Geometry: final body of the model. Coordinates: model frame, mm. A direction names the side the tool comes from. Give positions to 0.01 mm unless a question says otherwise; leave off trailing zeros. Order: outer loops, then holes, each group sorted by start corner. A loop starts at its lowest first (then second) coordinate and runs counter-clockwise, first axis right, second up. Notation, with made-up numbers: (17, 35) -> (26, 35) arc R12 cw to (26, 40) -> close; hole circle Ø1 at (61.5, -22). An arc over 180 degrees is marked (long way). Write item = value, one per line.
```python
from build123d import *

# Parameters (mm, degrees)
F0_W      = 32.2
F0_H      = 31.2
F1_DEPTH  = 4.2
F2_W      = 9.2
F2_H      = 8.6
F3_DEPTH  = 8.4
F2_W_2    = 25.4
F2_H_2    = 24.4
F4_DEPTH  = 4.5
F5_DEPTH  = 5
F2_W_3    = 17
F2_H_3    = 2
F6_DEPTH  = 4.1
F7_DEPTH  = 6.8
F8_R      = 2.5
F9_DEPTH  = 2
F10_R     = 2.5
F11_DEPTH = 2


with BuildPart() as f1:
    # F0 (on Front) → F1 (new body, symmetric)
    with BuildSketch(Plane.XZ):
        Rectangle(F0_W, F0_H)
    extrude(amount=F1_DEPTH, both=True)

    # F2 (on face) → F3 (cut, through all)
    with BuildSketch(Plane.XZ.offset(4.2)):
        with Locations((0, -2.8)):
            Rectangle(F2_W, F2_H)
    extrude(amount=-F3_DEPTH, mode=Mode.SUBTRACT)

    # F2 (on face) → F4 (cut)
    with BuildSketch(Plane.XZ.offset(4.2)):
        Polygon((14.1, -13.6), (14.1, 13.6), (-14.1, 13.6), (-14.1, -13.6), (-8.5, -13.6), (8.5, -13.6), align=None)
        Rectangle(F2_W_2, F2_H_2, mode=Mode.SUBTRACT)
    extrude(amount=-F4_DEPTH, mode=Mode.SUBTRACT)

    # F5 (cut): a face of the model
    f5_faces = [f1.faces().sort_by_distance(p)[0] for p in [
        (-12.3477898355, -4.2, 0),
    ]]
    extrude(f5_faces, amount=-F5_DEPTH, mode=Mode.SUBTRACT)

    # F2 (on face) → F6 (cut)
    with BuildSketch(Plane.XZ.offset(4.2)):
        with Locations((0, -14.6)):
            Rectangle(F2_W_3, F2_H_3)
    extrude(amount=-F6_DEPTH, mode=Mode.SUBTRACT)

    # F2 (on face) → F7 (cut)
    with BuildSketch(Plane.XZ.offset(4.2)):
        Polygon((-7.1, 1.5), (-4.6, 1.5), (4.6, 1.5), (7.1, 1.5), (7.1, 9.7), (-7.1, 9.7), align=None)
    extrude(amount=-F7_DEPTH, mode=Mode.SUBTRACT)

    # F8 (on face) → F9 (cut)
    with BuildSketch(Plane.YZ.offset(16.1)):
        with Locations((0, -10.6)):
            Circle(F8_R)
    extrude(amount=-F9_DEPTH, mode=Mode.SUBTRACT)

    # F10 (on face) → F11 (cut)
    with BuildSketch(Plane(origin=(-16.1, 0, 0), x_dir=(0, -1, 0), z_dir=(-1, 0, 0))):
        with Locations((0, -10.6)):
            Circle(F10_R)
    extrude(amount=-F11_DEPTH, mode=Mode.SUBTRACT)


solid = f1.part
```
1) Reachability of faces 4 (the face through (0, 2, 9.7)), 5 (the face through (0, -0.1, -15)), 6 (the face through (-4.6, 2, -3)) from +Z, -Z, +X, -X, +Y, -Y: full face, straight path, thin tool, end or side. Return the list, or none.
Check sheet entries:
face_4 = -Y
face_5 = -Z, -Y
face_6 = +Y, -Y
2) Section query C-C (z = -10.6). Output: boundary loops of the cut face in (x, y), plus the area to 3 significant figures.
Check sheet entries:
outline = (-16.1, -4.2) -> (-14.1, -4.2) -> (-14.1, -2.5) -> (-16.1, -2.5) -> close; (-16.1, 2.5) -> (-14.1, 2.5) -> (-14.1, 0.3) -> (-12.7, 0.3) -> (-12.7, 0.8) -> (12.7, 0.8) -> (12.7, 0.3) -> (14.1, 0.3) -> (14.1, 2.5) -> (16.1, 2.5) -> (16.1, 4.2) -> (-16.1, 4.2) -> close; (14.1, -4.2) -> (16.1, -4.2) -> (16.1, -2.5) -> (14.1, -2.5) -> close
area = 111 mm²
3) First-contact query: P1, Ø2, axis at x = 2.5, z = -14, coming from the -Y side; P2, Ø4, axis at y = 0, z = -10.6, coming from the -X side; P3, Ø2, axis at x = 0, z = 2, coming from the -Y side. Flat tips, straight axial feed; report the tip coordinate or a pass-through.
Check sheet entries:
P1 = -0.1
P2 = -14.1
P3 = 2.6
4) Section query B-B (x = 1). Output: boundary loops of the cut face in (y, z).
Check sheet entries:
outline = (-4.2, 13.6) -> (0.3, 13.6) -> (0.3, 12.2) -> (0.8, 12.2) -> (0.8, 9.7) -> (2.6, 9.7) -> (2.6, 1.5) -> (4.2, 1.5) -> (4.2, 15.6) -> (-4.2, 15.6) -> close; (-0.1, -15.6) -> (4.2, -15.6) -> (4.2, -7.1) -> (0.8, -7.1) -> (0.8, -12.2) -> (0.3, -12.2) -> (0.3, -13.6) -> (-0.1, -13.6) -> close
5) Line query: line 1 (Z direction, x = -15.4, y = 0); line 2 (Z direction, x = -3, y = 0.5); line 3 (X direction, y = 1.5, z = -4). Output: solid intervals per line, ascending. Write a range as from..to.
Check sheet entries:
line_1 = -15.6..-13.1, -8.1..15.6
line_2 = -15.6..-12.2, 12.2..15.6
line_3 = -16.1..-4.6, 4.6..16.1
6) Section query D-D (x = -13.5). Output: boundary loops of the cut face in (y, z), plus the area to 3 significant figures.
Check sheet entries:
outline = (-4.2, -15.6) -> (4.2, -15.6) -> (4.2, 15.6) -> (-4.2, 15.6) -> (-4.2, 13.6) -> (0.3, 13.6) -> (0.3, -13.6) -> (-4.2, -13.6) -> close
area = 140 mm²
7) Section query A-A (z = -1). Output: boundary loops of the cut face in (x, y).
Check sheet entries:
outline = (-16.1, -4.2) -> (-14.1, -4.2) -> (-14.1, 0.3) -> (-12.7, 0.3) -> (-12.7, 0.8) -> (-4.6, 0.8) -> (-4.6, 4.2) -> (-16.1, 4.2) -> close; (4.6, 0.8) -> (12.7, 0.8) -> (12.7, 0.3) -> (14.1, 0.3) -> (14.1, -4.2) -> (16.1, -4.2) -> (16.1, 4.2) -> (4.6, 4.2) -> close
8) Mould query, pull axis Z, two halves, no side actions, for faces 1 (the face through (0, 4.2, 4)), 2 (the face through (0, 0, 15.6)), 3 (the face through (4.6, 2, -3)). Classes: +Z half, -Z half, draft (parallel to the pull), parting line (faces both ways), or undercut.
Check sheet entries:
face_1 = draft
face_2 = +Z half
face_3 = undercut
